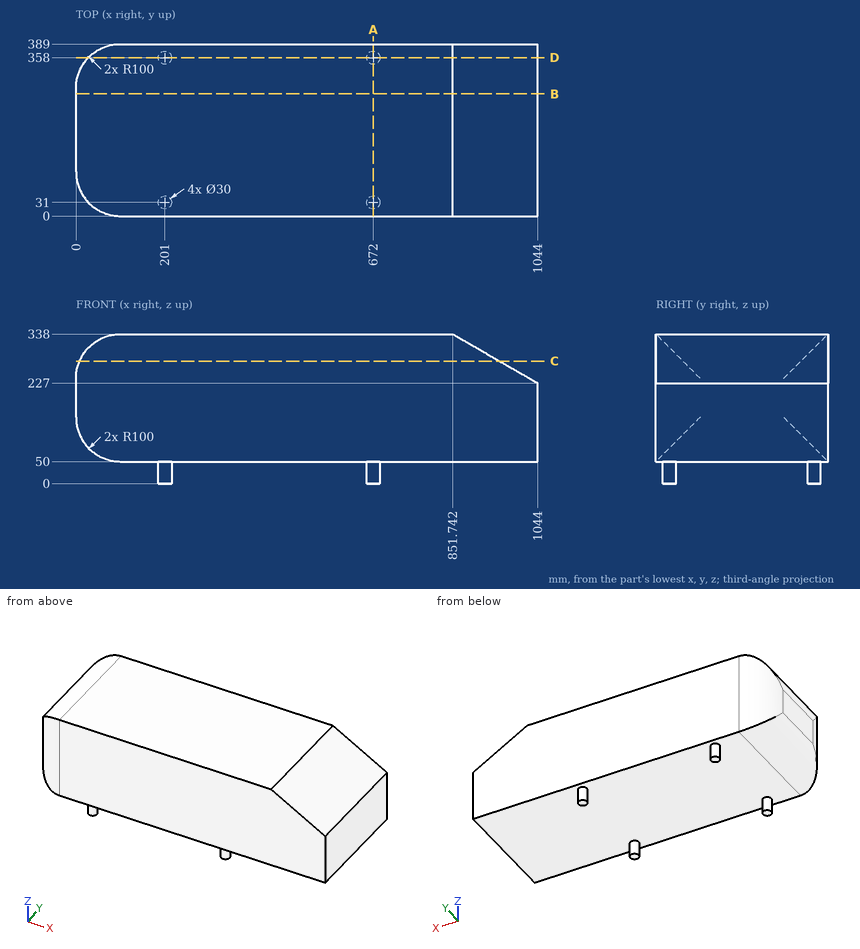
Print and shaded views of the part. All mm, measured from the part's lowest x, y and z. Round coordinates to 2 decimals unless told otherwise and drop trailing zeros. Write each loop counter-clockwise with the first axis right and the second up, starting at its lowest first coordinate (ties: lowest second). Pieces come first, ordered by that corner, then holes. Notation, with made-up numbers: (2, -21.75) - (46, -21.75) arc R12 cw to (46, -10.75) - close; hole circle Ø8 at (40, 27). An arc over 180 degrees is marked (long way). Write each question's results on one line, items separated by ' | '. Start each with the question number.
Item 1: Saw through at D-D (y = 358). Write the cut outline in (x, z).
Item 2: Drop flat-ended pins along their axis: P1, Ø4, axis at y = 192, z = 250.5, coming from the -X side; P2, Ø4, axis at x = 340, y = 185.5, coming from the -Z side; P3, Ø4, axis at y = 243, z = 232.5, coming from the -X side. Give the stop position or say it passes through.
Item 3: Saw through at B-B (y = 276). Write the cut outline in (x, z).
Item 4: Saw through at A-A (x = 672). Write the cut outline in (y, z).
Item 5: Saw through at C-C (z = 277). Write the cut outline in (x, y), and give its area (3 significant figures).
Item 6: Wall check: L1, parallel to Z at x = 513, y = 101.5; L2, parallel to X at y = 23, z = 48; L3, parallel to Z at x = 865, y = 171.5 (1 decimal). Give the ranges that are in metal, low to high. Write a range as [from, to].
Results are:
1) outline: (27.62, 81) arc R100 ccw to (100, 50) - (186, 50) - (186, 0) - (216, 0) - (216, 50) - (657, 50) - (657, 0) - (687, 0) - (687, 50) - (1044, 50) - (1044, 227) - (851.74, 338) - (100, 338) arc R100 ccw to (27.62, 307) - close
2) P1: stops at x = 0.55 | P2: stops at z = 50 | P3: stops at x = 0
3) outline: (0, 150) arc R100 ccw to (100, 50) - (1044, 50) - (1044, 227) - (851.74, 338) - (100, 338) arc R100 ccw to (0, 238) - close
4) outline: (0, 50) - (16, 50) - (16, 0) - (46, 0) - (46, 50) - (343, 50) - (343, 0) - (373, 0) - (373, 50) - (389, 50) - (389, 338) - (0, 338) - close
5) outline: (7.92, 61) arc R100 ccw to (100, 0) - (957.4, 0) - (957.4, 389) - (100, 389) arc R100 ccw to (7.92, 328) - close | area: 366,000 mm²
6) L1: z = [50, 338] | L2: x = [188.31, 213.69], [659.31, 684.69] | L3: z = [50, 330.3]
